Can you work these out from the model? Positions are in its coordinate system, mm. Face numbers are marked on the shaded views. A direction names the side the tool comes from. Coordinates: 2 decimals unless noted, no trailing zeros. Order: outer loops, then holes, each group sorted by start corner. A loop starts at its lowest first (then second) coordinate and runs counter-clockwise, first axis right, second up. Notation, with made-up numbers: (79, -40) - (111, -40) arc R21 ccw to (111, -17) - close; hole circle Ø1 at (85, 7). An arc over 180 degrees is marked (long way). Use a Markdown table: item, result. Add a question column.
(1) For pin 1 Ø1.5 at (x, z) = (1, -1.5) entering from +Y; pin 2 Ø2 at (y, z) = (-3, -3) entering from +X; pin 3 Ø2 at (x, z) = (3.5, -6.5) entering from +Y; pin 4 Ø6 at (y, z) = (-4.5, 0.5) entering from -X, each with a flat end and sliding along its axis, tell me the tip position at first contact or that it passes through.
(2) I want a section at B-B (z = 0). List the corners of the cut face in (x, y) for me.
(3) I want a section at A-A (y = 0). List the corners of the cut face in (x, z) for me, and give its area (3 significant figures).
(4) I want a section at C-C (x = 4.75). List the corners of the cut face in (y, z) for me.
(5) On a 3-axis mill with a long thin cutter (end or side, diameter ignored), from which of +Z, -Z, +X, -X, +Y, -Y can I reach the whole of each face in a straight line? I mean the marked faces 1, 2 and 3. Say none if no direction works.
(6) I want a section at D-D (x = 1.7). List the corners of the cut face in (y, z) for me.
(7) If I drill on L1, parallel to X at y = 3, z = -3; L2, parallel to Z at x = 1.65, y = -6.5; L3, parallel to Z at x = 2, y = 4.5, over which ranges is the centre line in solid material (lowest first)? Write a range as [from, to].
Solid Edge part; units mm, degrees
sketch "Sketch1" plane through (0, 0, 0) normal (0, -1, 0) x (1, 0, 0)
  line L0 (6, 2.5) -> (3, 2.5)
  line L1 (3, 2.5) -> (3, 8)
  line L2 (3, 8) -> (0, 8)
  line L3 (0, 8) -> (0, 0)
  line L4 (6, 0) -> (6, 2.5)
  dimension "D1" = 3
  dimension "D2" = 6
revolve "RevolvedProtrusion1" add sketch "Sketch1" angle 360 about axis through (0, 0, 0) along (1, 0, 0)
chamfer "Chamfer1" distance 0.2 angle 45 1 edges at (6, 0, -2.5)
sketch "Sketch2" plane through (6, 0, 0) normal (1, 0, 0) x (0, 1, 0)
  line L0 (-1.5, 2) -> (1.5, 2)
  arc A0 (1.5, 2) -> (-1.5, 2) centre (0, 0) cw
extrude "Extrusionsausschnitt_1" cut sketch "Sketch2" against normal blind 3 flip side to cut
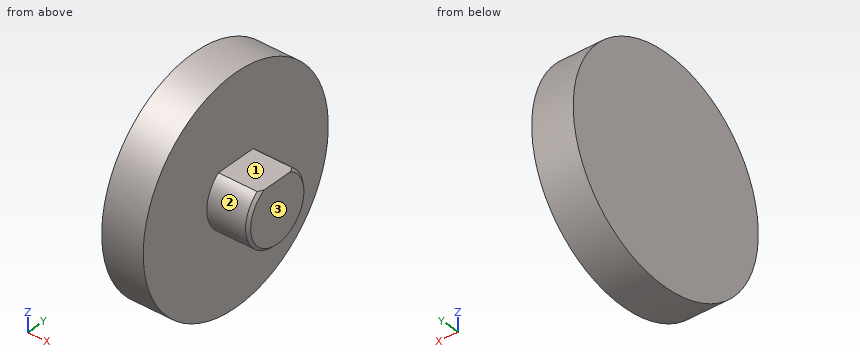
Answers follow:
| question | item | result |
|---|---|---|
| 1 | pin 1 | stops at y = 7.96 |
| 1 | pin 2 | stops at x = 3 |
| 1 | pin 3 | stops at y = 5.68 |
| 1 | pin 4 | stops at x = 0 |
| 2 | outline | (0, -8) - (3, -8) - (3, -2.5) - (5.8, -2.5) - (6, -2.3) - (6, 2.3) - (5.8, 2.5) - (3, 2.5) - (3, 8) - (0, 8) - close |
| 3 | outline | (0, -8) - (3, -8) - (3, -2.5) - (5.8, -2.5) - (6, -2.3) - (6, 2) - (3, 2) - (3, 8) - (0, 8) - close |
| 3 | area | 61.5 mm² |
| 4 | outline | (-1.5, 2) arc R2.5 ccw (long way) to (1.5, 2) - close |
| 5 | face 1 | +Z, +X, +Y, -Y |
| 5 | face 2 | +X |
| 5 | face 3 | +Z, -Z, +X, +Y, -Y |
| 6 | outline | circle Ø16 at (0, 0) |
| 7 | L1 | x = [0, 3] |
| 7 | L2 | z = [-4.66, 4.66] |
| 7 | L3 | z = [-6.61, 6.61] |
